Source: CAD feature listing. Evaluate the final solid. Frame: model axes, mm. A direction names the side the tool comes from. Coordinates: 2 decimals unless noted, no trailing zeros. Order: outer loops, then holes, each group sorted by start corner. A loop starts at its lowest first (then second) coordinate and runs counter-clockwise, first axis right, second up. Notation, with made-up numbers: (81, 27.25) -> (128, 27.25) arc R36 ccw to (128, 61.25) -> close; hole circle Ø5 at (-14, 44.25). An arc over 180 degrees is marked (long way). Put each result on its own line as item: value.
from build123d import *

# Parameters (mm, degrees)
RESSALTO_EXTRUS_O1_DEPTH  = 4.5
ESBO_O2_R                 = 5.1
CORTE_EXTRUS_O1_DEPTH     = 3.5
ESBO_O3_R                 = 3
CORTE_EXTRUS_O2_DEPTH     = 3.5
ESPELHAR2_COPY_1_DEPTH    = 4.5
ESPELHAR2_COPY_2_SKETCH_R = 5.1
ESPELHAR2_COPY_2_DEPTH    = 3.5
ESPELHAR2_COPY_3_SKETCH_R = 3
ESPELHAR2_COPY_3_DEPTH    = 3.5
ESBO_O5_W                 = 18
ESBO_O5_H                 = 14
RESSALTO_EXTRUS_O2_DEPTH  = 4.5
ESBO_O6_R                 = 5.15
CORTE_EXTRUS_O3_DEPTH     = 3.5
ESBO_O7_R                 = 3
CORTE_EXTRUS_O4_DEPTH     = 3.5
FILETE1_R                 = 10
ESBO_O8_W                 = 8.485281374
ESBO_O8_H                 = 8
ESBO_O8_W_2               = 12.985281374
RESSALTO_EXTRUS_O3_DEPTH  = 3.5


with BuildPart() as part:
    # Esboço1 → Ressalto-extrusão1 (new body)
    with BuildSketch(Plane.XY):
        Polygon((-8.485281374, 0), (-20, 11.514718626), (-20, 20), (-11.514718626, 20), (0, 8.485281374), (0, 0), align=None)
    ressalto_extrus_o1 = extrude(amount=RESSALTO_EXTRUS_O1_DEPTH)

    # Esboço2 → Corte-extrusão1 (cut)
    with BuildSketch(Plane.XY.offset(4.5)):
        with Locations((-13, 13)):
            Circle(ESBO_O2_R)
    corte_extrus_o1 = extrude(amount=-CORTE_EXTRUS_O1_DEPTH, mode=Mode.SUBTRACT)

    # Esboço3 → Corte-extrusão2 (cut)
    with BuildSketch(Plane.XY.offset(1)):
        with Locations((-13, 13)):
            Circle(ESBO_O3_R)
    corte_extrus_o2 = extrude(amount=-CORTE_EXTRUS_O2_DEPTH, mode=Mode.SUBTRACT)

    # Espelhar1: Ressalto-extrusão1, Corte-extrusão1, Corte-extrusão2 across plane
    add(ressalto_extrus_o1.mirror(Plane(origin=(0, 0, 0), x_dir=(0, 0, 1), z_dir=(1, 0, 0))))
    add(corte_extrus_o1.mirror(Plane(origin=(0, 0, 0), x_dir=(0, 0, 1), z_dir=(1, 0, 0))), mode=Mode.SUBTRACT)
    add(corte_extrus_o2.mirror(Plane(origin=(0, 0, 0), x_dir=(0, 0, 1), z_dir=(1, 0, 0))), mode=Mode.SUBTRACT)

    # Espelhar2: Ressalto-extrusão1, Corte-extrusão1, Corte-extrusão2 across plane
    add(ressalto_extrus_o1.mirror(Plane.ZX))
    add(corte_extrus_o1.mirror(Plane.ZX), mode=Mode.SUBTRACT)
    add(corte_extrus_o2.mirror(Plane.ZX), mode=Mode.SUBTRACT)

    # Espelhar2 copy 1 sketch → Espelhar2 copy 1 (add)
    with BuildSketch(Plane(origin=(0, 0, 0), x_dir=(-1, 0, 0), z_dir=(0, 0, 1))):
        Polygon((-8.485281374, 0), (-20, 11.514718626), (-20, 20), (-11.514718626, 20), (0, 8.485281374), (0, 0), align=None)
    extrude(amount=ESPELHAR2_COPY_1_DEPTH)

    # Espelhar2 copy 2 sketch → Espelhar2 copy 2 (cut)
    with BuildSketch(Plane(origin=(0, 0, 4.5), x_dir=(-1, 0, 0), z_dir=(0, 0, 1))):
        with Locations((-13, 13)):
            Circle(ESPELHAR2_COPY_2_SKETCH_R)
    extrude(amount=-ESPELHAR2_COPY_2_DEPTH, mode=Mode.SUBTRACT)

    # Espelhar2 copy 3 sketch → Espelhar2 copy 3 (cut)
    with BuildSketch(Plane(origin=(0, 0, 1), x_dir=(-1, 0, 0), z_dir=(0, 0, 1))):
        with Locations((-13, 13)):
            Circle(ESPELHAR2_COPY_3_SKETCH_R)
    extrude(amount=-ESPELHAR2_COPY_3_DEPTH, mode=Mode.SUBTRACT)

    # Esboço5 → Ressalto-extrusão2 (add)
    with BuildSketch(Plane(origin=(20, 0, 0), x_dir=(0, 0, -1), z_dir=(1, 0, 0))):
        with Locations((-9, 13)):
            Rectangle(ESBO_O5_W, ESBO_O5_H)
    ressalto_extrus_o2 = extrude(amount=RESSALTO_EXTRUS_O2_DEPTH)

    # Esboço6 → Corte-extrusão3 (cut)
    with BuildSketch(Plane.ZY.offset(-20)):
        with Locations((11.5, 13)):
            Circle(ESBO_O6_R)
    corte_extrus_o3 = extrude(amount=-CORTE_EXTRUS_O3_DEPTH, mode=Mode.SUBTRACT)

    # Esboço7 → Corte-extrusão4 (cut)
    with BuildSketch(Plane.ZY.offset(-23.5)):
        with Locations((11.5, 13)):
            Circle(ESBO_O7_R)
    corte_extrus_o4 = extrude(amount=-CORTE_EXTRUS_O4_DEPTH, mode=Mode.SUBTRACT)

    # Espelhar3: Ressalto-extrusão2, Corte-extrusão3, Corte-extrusão4 across plane
    add(ressalto_extrus_o2.mirror(Plane.ZX))
    add(corte_extrus_o3.mirror(Plane.ZX), mode=Mode.SUBTRACT)
    add(corte_extrus_o4.mirror(Plane.ZX), mode=Mode.SUBTRACT)

    # Filete1
    # the kernel refuses this fillet: 10 mm, written as the material it adds along each edge
    with BuildSketch(Plane(origin=(20, 11.514718626, 0), x_dir=(0, -1, 0), z_dir=(0, 0, 1))) as filete1_piece_1:
        with BuildLine():
            CenterArc((15.431276309, -1.289140686), FILETE1_R, 172.593154991, 52.406845009)
            Line((8.360208498, -8.360208498), (0, 0))
            Line((0, 0), (5.514718626, 0))
        make_face()
    extrude(amount=4.5)
    with BuildSketch(Plane(origin=(20, -11.514718626, 0), x_dir=(-0.7071067811865462, 0.7071067811865488, 0), z_dir=(0, 0, 1))) as filete1_piece_2:
        with BuildLine():
            CenterArc((11.823120241, -10), FILETE1_R, 90, 52.406845009)
            Line((3.899494937, -3.899494937), (0, 0))
            Line((0, 0), (11.823120241, 0))
        make_face()
    extrude(amount=4.5)

    # Esboço8 → Ressalto-extrusão3 (add)
    with BuildSketch(Plane(origin=(0, 20, 0), x_dir=(1, 0, 0), z_dir=(0, 1, 0))):
        with Locations((-15.757359313, -4)):
            Rectangle(ESBO_O8_W, ESBO_O8_H)
        with Locations((18.007359313, -4)):
            Rectangle(ESBO_O8_W_2, ESBO_O8_H)
    extrude(amount=RESSALTO_EXTRUS_O3_DEPTH)


solid = part.part
1. Cut plane D-D on x = -3.5. Output: boundary loops of the cut face in (y, z).
Numbers:
outline: (-11.99, 0) -> (11.99, 0) -> (11.99, 4.5) -> (-11.99, 4.5) -> close
2. Cut plane C-C on y = -13. Count the separate pieces of the cut face and the enclosed holes in it, plus the area to 3 significant figures.
Numbers:
separate pieces: 5
enclosed holes: 0
area: 94.9 mm2
3. First-contact query: pin 1 (9 mm diameter, centred on x = 13, y = -13, fed in from +Z); pin 2 (8 mm diameter, centred on y = -8, z = 12.5, fed in from -X); pin 3 (5 mm diameter, centred on x = 11.5, y = -15.5, fed in from +Z). Flat tips, straight axial feed; report the tip coordinate or a pass-through.
Numbers:
pin 1: stops at z = 1
pin 2: stops at x = 20
pin 3: stops at z = 4.5
4. Pull-direction query (X, two-part tool) for faces 1 (the flat face through (0, 0, 4.5)), 2 (the flat face through (-20, -16, 2)), 3 (the flat face through (24.5, -13, 7)), 4 (the flat face through (-9.7, -13.1, 1)); classes: pulls with the +X half, pulls with the -X half, needs draft (parallel to the pull), parting line crosses it, or undercut.
Numbers:
face 1: needs draft
face 2: pulls with the -X half
face 3: pulls with the +X half
face 4: undercut
5. Ray query, line 1 along Y through (x, z) = (24.1, 11.5); line 2 along X through (y, z) = (-17, 1.75); line 3 along X through (y, z) = (12.5, 1.25). Return the intervals inside material, ascending.
Numbers:
line 1: y = -20 to -16, -10 to -6, 6 to 10, 16 to 20
line 2: x = -20 to -16.16, -9.84 to -8.51, 8.51 to 9.84, 16.16 to 24.5
line 3: x = -20 to -18.08, -7.92 to -4.01, 4.01 to 7.92, 18.08 to 24.5
6. Cut plane B-B on x = 14. Output: boundary loops of the cut face in (y, z).
Numbers:
outline: (-20, 0) -> (-15.83, 0) -> (-15.83, 1) -> (-18, 1) -> (-18, 4.5) -> (-20, 4.5) -> close; (-10.17, 0) -> (-4.9, 0) -> (-4.9, 4.5) -> (-8, 4.5) -> (-8, 1) -> (-10.17, 1) -> close; (4.9, 0) -> (10.17, 0) -> (10.17, 1) -> (8, 1) -> (8, 4.5) -> (4.9, 4.5) -> close; (15.83, 0) -> (23.5, 0) -> (23.5, 8) -> (20, 8) -> (20, 4.5) -> (18, 4.5) -> (18, 1) -> (15.83, 1) -> close
7. Cut plane A-A on z = 11.5. Output: boundary loops of the cut face in (x, y), plus the area to 3 significant figures.
Numbers:
outline: (20, -20) -> (24.5, -20) -> (24.5, -16) -> (23.5, -16) -> (23.5, -18.15) -> (20, -18.15) -> close; (20, -7.85) -> (23.5, -7.85) -> (23.5, -10) -> (24.5, -10) -> (24.5, -6) -> (20, -6) -> close; (20, 6) -> (24.5, 6) -> (24.5, 10) -> (23.5, 10) -> (23.5, 7.85) -> (20, 7.85) -> close; (20, 18.15) -> (23.5, 18.15) -> (23.5, 16) -> (24.5, 16) -> (24.5, 20) -> (20, 20) -> close
area: 41.9 mm2
8. Set-up query: faces 5 (the cylindrical face through (21.73, -14.55, 16.41)), 6 (the cylindrical face through (8.289, 11.047, 2.774)), 7 (the flat face through (22, 20, 13)). Return all of +Z, -Z, +X, -X, +Y, -Y with unobstructed straight access to the full face (end or side cutting, diameter ignored); none if empty.
Numbers:
face 5: -X
face 6: +Z
face 7: +Z, +X, -X, +Y
